from build123d import *

# Parameters (mm, degrees)
BOSS_EXTRUDE1_DEPTH   = 6.35
CUT_EXTRUDE1_DEPTH    = 6.35
SKETCH5_R             = 1.5875
CUT_EXTRUDE4_DEPTH    = 7.62
SKETCH7_R             = 0.24003
CUT_EXTRUDE5_DEPTH    = 22.717
F_2_56_TAPPED_HOLE1_D = 1.778


with BuildPart() as part:
    # Sketch1 → Boss-Extrude1 (new body)
    with BuildSketch(Plane.XY):
        Polygon((0, 0), (12.192, 0), (12.192, -4.064), (17.526, -11.557), (17.526, -21.717), (8.382, -21.717), (8.382, -11.557), (3.048, -4.064), (0, -4.064), align=None)
    extrude(amount=-BOSS_EXTRUDE1_DEPTH)

    # Sketch2 → Cut-Extrude1 (cut)
    with BuildSketch(Plane(origin=(0, 0, 0), x_dir=(1, 0, 0), z_dir=(0, 1, 0))):
        with BuildLine():
            Line((1.27, 6.35), (-1.332869865, 6.35))
            Line((-1.332869865, 6.35), (-1.332869865, 0))
            Line((-1.332869865, 0), (1.27, 0))
            ThreePointArc((1.27, 0), (0, 3.175), (1.27, 6.35))
        make_face()
    extrude(amount=-CUT_EXTRUDE1_DEPTH, mode=Mode.SUBTRACT)

    # Sketch5 → Cut-Extrude4 (cut)
    with BuildSketch(Plane.XZ.offset(21.717)):
        with Locations((12.954, -3.175)):
            Circle(SKETCH5_R)
    extrude(amount=-CUT_EXTRUDE4_DEPTH, mode=Mode.SUBTRACT)

    # Sketch7 → Cut-Extrude5 (cut, through all)
    with BuildSketch(Plane(origin=(0, 0, 0), x_dir=(1, 0, 0), z_dir=(0, 1, 0))):
        with Locations((0.54102, 3.175)):
            Circle(SKETCH7_R)
    extrude(amount=-CUT_EXTRUDE5_DEPTH, mode=Mode.SUBTRACT)

    # #2-56 Tapped Hole1 (through all)
    with Locations(Plane(origin=(12.192, 0, 0), x_dir=(0, 0, -1), z_dir=(1, 0, 0))):
        with Locations((3.175, -2.032)):
            Hole(F_2_56_TAPPED_HOLE1_D / 2)


solid = part.part
Geometry: final body of the model. Coordinates: model frame, mm. A direction names the side the tool comes from. Coordinates: 2 decimals unless noted, no trailing zeros. Order: outer loops, then holes, each group sorted by start corner. A loop starts at its lowest first (then second) coordinate and runs counter-clockwise, first axis right, second up. Notation, with made-up numbers: (18.5, 87) - (53.5, 87) arc R16 cw to (53.5, 103) - close; hole circle Ø5 at (41, -15). An arc over 180 degrees is marked (long way). Use one line per item in the form item = value.
1) Section B-B (z = -1.25). Return loops of the section in (x, y), then the cut area to 3 significant figures.
Solutions:
outline = (0.42, -4.06) - (3.05, -4.06) - (8.38, -11.56) - (8.38, -21.72) - (17.53, -21.72) - (17.53, -11.56) - (12.19, -4.06) - (12.19, 0) - (0.42, 0) - close
area = 209 mm^2
2) Set-up query: faces 1 (the face through (11, -11, -6.35)), 2 (the face through (17.526, -17, -3)), 3 (the face through (8.382, -17, -3)), 4 (the face through (13, -14.097, -3)), 5 (the face through (12.192, -2, -2)). Return all of +Z, -Z, +X, -X, +Y, -Y with unobstructed straight access to the full face (end or side cutting, diameter ignored); none if empty.
Solutions:
face_1 = -Z, +X, -X, +Y, -Y
face_2 = +Z, -Z, +X, +Y, -Y
face_3 = +Z, -Z, -X, -Y
face_4 = -Y
face_5 = +Z, -Z, +X, +Y
3) Pin query (flat end, axial travel): pin 1 (1.9 mm diameter, centred on y = -15.5, z = -3.5, fed in from -X); pin 2 (3 mm diameter, centred on x = 5.5, z = -1, fed in from -Y); pin 3 (1.6 mm diameter, centred on x = 13.5, z = -3, fed in from -Y). Return the tip coordinate at first contact, or that it passes through.
Solutions:
pin_1 = 8.38
pin_2 = -9.62
pin_3 = -14.1
4) Section D-D (x = 12.5). Return loops of the section in (y, z), then the cut area to 3 significant figures.
Solutions:
outline = (-21.72, -6.35) - (-4.5, -6.35) - (-4.5, 0) - (-21.72, 0) - (-21.72, -1.65) - (-14.1, -1.65) - (-14.1, -4.7) - (-21.72, -4.7) - close
area = 86.2 mm^2
5) Ray query, L1, parallel to X at y = -15.75, z = -1.5; L2, parallel to Y at x = 7.75, z = -3; L3, parallel to Z at x = 12.5, y = -17. Return the intervals inside material, ascending.
Solutions:
L1 = 8.38 to 17.53
L2 = -10.67 to -2.9, -1.16 to 0
L3 = -6.35 to -4.7, -1.65 to 0
6) Mould query, pull axis Z, two halves, no side actions, for faces 6 (the face through (5.75, -7.86, -3.13)), 7 (the face through (14.42, -17.96, -3.78)), 8 (the face through (0.074, -1.1, -2.352)). Classes: +Z half, -Z half, draft (parallel to the pull), parting line (faces both ways), or undercut.
Solutions:
face_6 = draft
face_7 = undercut
face_8 = parting line
7) Section A-A (x = 10.25). Return loops of the section in (y, z) (3 decimals).
Solutions:
outline = (-21.717, -6.35) - (0, -6.35) - (0, 0) - (-21.717, 0) - close; hole circle Ø1.778 at (-2.032, -3.175)
